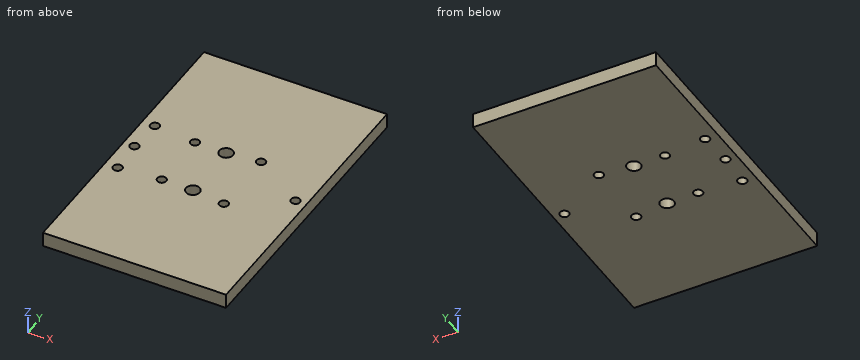
Autodesk Inventor part; units mm, degrees
ref_plane "YZ Plane" through (0, 0, 0) normal (1, 0, 0) x (0, 1, 0)
ref_plane "XZ Plane" through (0, 0, 0) normal (0, 1, 0) x (-1, 0, 0)
ref_plane "XY Plane" through (0, 0, 0) normal (0, 0, 1) x (1, 0, 0)
sketch "Sketch1" plane through (0, 0, 0) normal (0, 0, 1) x (1, 0, 0)
  circle A0 centre (50, 45.5) radius 2.5
  circle A1 centre (-8, 45.5) radius 2.5
  circle A2 centre (32, 43.5) radius 3.75
  circle A3 centre (15, 43.5) radius 2.4585
  line L0 (57, 54) -> (-15, 54)
  line L1 (-15, 54) -> (-15, 37)
  line L2 (57, 37) -> (-15, 37)
  line L3 (57, 54) -> (57, 37)
  circle A4 centre (50, 8.5) radius 2.5
  circle A5 centre (-8, 8.5) radius 2.5
  circle A6 centre (32, 10.5) radius 3.75
  circle A7 centre (15, 10.5) radius 2.4585
  line L4 (57, 0) -> (-15, 0)
  line L5 (57, 0) -> (57, 17)
  line L6 (57, 17) -> (-15, 17)
  line L7 (-15, 0) -> (-15, 17)
  line L8 (-15, 107) -> (85, 107)
  line L9 (85, 107) -> (85, -53)
  line L10 (85, -53) -> (-15, -53)
  line L11 (-15, -53) -> (-15, 107)
  line L12 (-94.8305, 27) -> (141.7075, 27) construction
  circle A8 centre (-9, 27) radius 2.5
  circle A9 centre (79, 27) radius 2.5
  point P0 (0, 0)
  point P1 (52.2653, 16.3)
  dimension "d0" = 100
  dimension "d1" = 160
  dimension "d2" = 20
  dimension "d3" = 10
  dimension "d4" = 72
  dimension "d5" = 0
  dimension "d6" = 80
  dimension "d7" = 5
  dimension "d8" = 5
  dimension "d9" = 6
  dimension "d10" = 6
extrude "Extrusion1" add sketch "Sketch1" along normal blind 8
equation "\"d3\" = 0.5 * d2"
equation "\"d6\" = 0.5 * d1"
properties part number "spool main support"
Verification items for the finished model (mm, model axes). Coordinates: 2 decimals unless noted, no trailing zeros. Write each loop counter-clockwise with the first axis right and the second up, starting at its lowest first coordinate (ties: lowest second). Pieces come first, ordered by that corner, then holes. Notation, with made-up numbers: M -27,87.5 L 27,87.5 A21 cw 27,118.5 Z; hole C 6,34.25 d2. An arc over 180 degrees is marked long. Answer as a JSON object with one key per item and string values. Group by question number.
(1) Material ranges on line 1 (Y direction, x = 32, z = 5); line 2 (Y direction, x = 15, z = 4.5); line 3 (Y direction, x = 79, z = 3.5), recorded low to high.
(2) Gauge pin test, flat end, axial feed: pin 1 (7 mm diameter, centred on x = 32, y = 43.5, fed in from -Z). Record the tip position at first contact, or that the pin passes through.
(3) Cross-section at B-B, the plane z = 6. State how many separate pieces and enclosed holes the cut face has, and give its area (3 significant figures).
(4) Cross-section at A-A, the plane x = 32. Record the cut outline in (y, z).
Reply:
{
 "1": {"line 1": "-53 to 6.75, 14.25 to 39.75, 47.25 to 107", "line 2": "-53 to 8.04, 12.96 to 41.04, 45.96 to 107", "line 3": "-53 to 24.5, 29.5 to 107"},
 "2": {"pin 1": "through"},
 "3": {"separate pieces": "1", "enclosed holes": "10", "area": "15,800 mm²"},
 "4": {"outline": "M -53,0 L 6.75,0 L 6.75,8 L -53,8 Z; M 14.25,0 L 39.75,0 L 39.75,8 L 14.25,8 Z; M 47.25,0 L 107,0 L 107,8 L 47.25,8 Z"}
}
